Part model, mm, in its own coordinate system. A direction names the side the tool comes from. Round coordinates to 2 decimals unless told otherwise and drop trailing zeros. Return JSON: item names as keys, results as strings. Group by question number.
Item 1: Probe probe 1 along Y at (x, z) = (39.5, 5.5) (1 decimal); probe 2 along X at (y, z) = (-10, 8); probe 3 along Y at (x, z) = (-10, 9.25) (1 decimal). List the from-to ranges inside material, lowest first.
Item 2: Drop flat-ended pins along their axis: pin 1 (0.8 mm diameter, centred on y = -7.5, z = 6, fed in from -X); pin 2 (3 mm diameter, centred on y = 0.5, z = 3, fed in from -X) (3 decimals); pin 3 (5 mm diameter, centred on x = 65, z = 6.5, fed in from +Y). Give the stop position or say it passes through.
Item 3: Saw through at A-A on y = 0. State how many separate pieces and enclosed holes the cut face has, and give its area (3 significant figures).
Item 4: Tool access for faces 5 (the face through (11, -9.525, 5)), 6 (the face through (62.386, 0.715, 2.491)), 7 (the face through (-27, 0, 0)): list every direction of +Z, -Z, +X, -X, +Y, -Y with a clear straight run to the whole face (end or side of a thin tool).
Item 5: Two-plate mould, pull along Y, no slides. Class faces 1 (the face through (15.15, 0.1, 4.83)), 2 (the face through (-27, 0, 9.525)), 3 (the face through (-56.214, 0.57, 4.696)), 4 (the face through (7, -12.7, 5)): released by +Y, released by -Y, zero draft, split by the parting line, or undercut.
```python
from build123d import *

# Parameters (mm, degrees)
SKETCH1_R           = 4
BOSS_EXTRUDE1_DEPTH = 9.525
SKETCH3_R           = 1.89865
SKETCH3_R_2         = 1.9939
CUT_EXTRUDE2_DEPTH  = 10.525
SKETCH19_W          = 13.97
SKETCH19_H          = 3.556
CUT_EXTRUDE4_DEPTH  = 10.525
CUT_EXTRUDE5_REACH  = 168.05
SKETCH20_R          = 2.38125
FILLET5_R           = 5.08
FILLET6_R           = 5.08
FILLET7_R           = 1.27


with BuildPart() as part:
    # Sketch1 → Boss-Extrude1 (new body)
    with BuildSketch(Plane.XY):
        with BuildLine():
            Line((73.025, 12.7), (73.025, -12.7))
            Line((73.025, -12.7), (-57.574757283, -12.7))
            ThreePointArc((-57.574757283, -12.7), (-64.480996255, -18.08314132), (-73.025, -20))
            ThreePointArc((-73.025, -20), (-93.025, 0), (-73.025, 20))
            ThreePointArc((-73.025, 20), (-64.480996255, 18.08314132), (-57.574757283, 12.7))
            Line((-57.574757283, 12.7), (73.025, 12.7))
        make_face()
        with Locations((-73.025, 0)):
            Circle(SKETCH1_R, mode=Mode.SUBTRACT)
    extrude(amount=BOSS_EXTRUDE1_DEPTH)

    # Sketch3 → Cut-Extrude2 (cut, through all)
    with BuildSketch(Plane.XY):
        with Locations((-73.025, 15)):
            Circle(SKETCH3_R)
        with Locations((-58.025, 0)):
            Circle(SKETCH3_R)
        with Locations((-73.025, -15)):
            Circle(SKETCH3_R)
        with Locations((-88.025, 0)):
            Circle(SKETCH3_R)
        with Locations((-83.631601718, -10.606601718)):
            Circle(SKETCH3_R_2)
        with Locations((-83.631601718, 10.606601718)):
            Circle(SKETCH3_R_2)
        with Locations((-62.418398282, 10.606601718)):
            Circle(SKETCH3_R_2)
        with Locations((-62.418398282, -10.606601718)):
            Circle(SKETCH3_R_2)
    extrude(amount=CUT_EXTRUDE2_DEPTH, mode=Mode.SUBTRACT)

    # Sketch19 → Cut-Extrude4 (cut, through all)
    with BuildSketch(Plane.XY.offset(9.525)):
        Polygon((-51.4245, -9.525), (-32.3745, -9.525), (-51.4245, 9.525), align=None)
        with Locations((62.2405, 7.747)):
            Rectangle(SKETCH19_W, SKETCH19_H)
        Polygon((-47.6145, 9.525), (-28.5645, -9.525), (-28.5645, 9.525), align=None)
        Polygon((-1.8945, -9.525), (-20.9445, -9.525), (-1.8945, 9.525), align=None)
        Polygon((-24.7545, -9.525), (-24.7545, 9.525), (-5.7045, 9.525), align=None)
        Polygon((1.9155, -9.525), (1.9155, 9.525), (20.9655, -9.525), align=None)
        Polygon((5.7255, 9.525), (24.7755, -9.525), (24.7755, 9.525), align=None)
        Polygon((28.5855, 9.525), (47.6355, 9.525), (28.5855, -9.525), align=None)
        Polygon((51.4455, -9.525), (32.3955, -9.525), (51.4455, 9.525), align=None)
        with Locations((62.2405, -7.747)):
            Rectangle(SKETCH19_W, SKETCH19_H)
    extrude(amount=-CUT_EXTRUDE4_DEPTH, mode=Mode.SUBTRACT)

    # Sketch20 → Cut-Extrude5 (cut, up to next)
    with BuildSketch(Plane(origin=(73.025, 0, 0), x_dir=(0, 0, -1), z_dir=(1, 0, 0)), mode=Mode.PRIVATE) as cut_extrude5_sk1:
        with Locations((-4.7625, 0)):
            Circle(SKETCH20_R)
    cut_extrude5_tool1 = extrude(cut_extrude5_sk1.sketch, amount=-CUT_EXTRUDE5_REACH, mode=Mode.PRIVATE) & part.part
    add(cut_extrude5_tool1.solids().sort_by_distance((73.025, 0, 4.7625))[0], mode=Mode.SUBTRACT)

    # Fillet5
    fillet5_edges = [part.edges().sort_by_distance(p)[0] for p in [
        (73.025, 12.7, 4.7625),
        (73.025, -12.7, 4.7625),
    ]]
    fillet(fillet5_edges, radius=FILLET5_R)

    # Fillet6
    fillet6_edges = [part.edges().sort_by_distance(p)[0] for p in [
        (-57.574757283, 12.7, 4.7625),
        (-57.574757283, -12.7, 4.7625),
    ]]
    fillet(fillet6_edges, radius=FILLET6_R)

    # Fillet7
    fillet7_edges = [part.edges().sort_by_distance(p)[0] for p in [
        (51.4455, 9.525, 4.7625),
        (51.4455, -9.525, 4.7625),
        (32.3955, -9.525, 4.7625),
        (69.2255, -9.525, 4.7625),
        (55.2555, -9.525, 4.7625),
        (55.2555, -5.969, 4.7625),
        (69.2255, -5.969, 4.7625),
        (-51.4245, 9.525, 4.7625),
        (-32.3745, -9.525, 4.7625),
        (-51.4245, -9.525, 4.7625),
        (20.9655, -9.525, 4.7625),
        (1.9155, -9.525, 4.7625),
        (1.9155, 9.525, 4.7625),
        (-5.7045, 9.525, 4.7625),
        (-24.7545, -9.525, 4.7625),
        (-24.7545, 9.525, 4.7625),
        (-1.8945, 9.525, 4.7625),
        (-1.8945, -9.525, 4.7625),
        (-20.9445, -9.525, 4.7625),
        (55.2555, 5.969, 4.7625),
        (55.2555, 9.525, 4.7625),
        (69.2255, 9.525, 4.7625),
        (69.2255, 5.969, 4.7625),
        (-47.6145, 9.525, 4.7625),
        (-28.5645, 9.525, 4.7625),
        (-28.5645, -9.525, 4.7625),
        (5.7255, 9.525, 4.7625),
        (24.7755, 9.525, 4.7625),
        (24.7755, -9.525, 4.7625),
        (28.5855, -9.525, 4.7625),
        (28.5855, 9.525, 4.7625),
        (47.6355, 9.525, 4.7625),
    ]]
    fillet(fillet7_edges, radius=FILLET7_R)


solid = part.part
```
Filled in:
{
 "1": {"probe 1": "y = -12.7 to -9.5, -2.4 to 1.4, 9.5 to 12.7", "probe 2": "x = -90.35 to -85.53, -81.73 to -64.32, -60.52 to 72.43", "probe 3": "y = -12.7 to -9.5, 1.4 to 5.2, 9.5 to 12.7"},
 "2": {"pin 1": "stops at x = -91.72", "pin 2": "stops at x = -93.025", "pin 3": "stops at y = 12.7"},
 "3": {"separate pieces": "13", "enclosed holes": "0", "area": "605 mm^2"},
 "4": {"face 5": "+Z, -Z", "face 6": "+X", "face 7": "-Z, +X, -X, +Y, -Y"},
 "5": {"face 1": "undercut", "face 2": "zero draft", "face 3": "undercut", "face 4": "released by -Y"}
}
